Input: part model. Units: mm. Frame: model coordinates. A direction names the side the tool comes from. Give positions to 0.01 mm unless a question says otherwise; leave off trailing zeros. Loops run counter-clockwise (first coordinate to the right, second up) from the corner with the lowest first, then second, coordinate; pieces in that order, holes last. Notation, with made-up numbers: (80.5, -7) -> (139.5, -7) arc R30 cw to (139.5, 24) -> close; hole circle Ø6 at (87.5, 62.5). An arc over 180 degrees is marked (long way). Answer as a JSON object with one key per item and string values.
```python
from build123d import *

# Parameters (mm, degrees)
F0_W     = 50
F0_H     = 100
F1_DEPTH = 2
F2_W     = 8
F2_H     = 20
F3_DEPTH = 10
F4_W     = 4
F4_H     = 36.223298
F5_DEPTH = 10


with BuildPart() as f1:
    # F0 (on Front) → F1 (new body)
    with BuildSketch(Plane.XZ):
        Rectangle(F0_W, F0_H)
    extrude(amount=F1_DEPTH)

    # F2 (on face) → F3 (join)
    with BuildSketch(Plane(origin=(0, 0, 0), x_dir=(-1, 0, 0), z_dir=(0, 1, 0))):
        Rectangle(F2_W, F2_H)
    extrude(amount=F3_DEPTH)

    # F4 (on face) → F5 (cut)
    with BuildSketch(Plane(origin=(0, 10, 0), x_dir=(-1, 0, 0), z_dir=(0, 1, 0))):
        Rectangle(F4_W, F4_H)
    extrude(amount=-F5_DEPTH, mode=Mode.SUBTRACT)


solid = f1.part
```
Q1. Section C-C, the plane x = -9. Return the cut outline in (y, z).
Evaluation:
{"outline": "(-2, -50) -> (0, -50) -> (0, 50) -> (-2, 50) -> close"}
Q2. Section A-A, the plane y = 7.5. Return the cut outline in (x, z).
Evaluation:
{"outline": "(-4, -10) -> (-2, -10) -> (-2, 10) -> (-4, 10) -> close; (2, -10) -> (4, -10) -> (4, 10) -> (2, 10) -> close"}
Q3. Access query for faces 4 (the flat face through (-3, 5, -10)), 5 (the flat face through (-4, 5, 0)), 6 (the flat face through (3, 5, 10)), 7 (the flat face through (4, 5, 0)), 8 (the flat face through (2, 5, 0)). Directions: +Z, -Z, +X, -X, +Y, -Y. A direction counts if a zero-diameter tool reaches every point of the face in a straight line with its end or side. Return the directions, or none.
Evaluation:
{"face 4": "-Z, +X, -X, +Y", "face 5": "+Z, -Z, -X, +Y", "face 6": "+Z, +X, -X, +Y", "face 7": "+Z, -Z, +X, +Y", "face 8": "+Z, -Z, +Y"}
Q4. Ray query, line 1 along X through (y, z) = (9.25, 3.5); line 2 along Y through (x, z) = (-7, -16); line 3 along Z through (x, y) = (-3.5, 8.5). Return the intervals inside material, ascending.
Evaluation:
{"line 1": "x = -4 to -2, 2 to 4", "line 2": "y = -2 to 0", "line 3": "z = -10 to 10"}
Q5. Section B-B, the plane z = 0. Return the cut outline in (x, y), then the cut area to 3 significant figures.
Evaluation:
{"outline": "(-25, -2) -> (25, -2) -> (25, 0) -> (4, 0) -> (4, 10) -> (2, 10) -> (2, 0) -> (-2, 0) -> (-2, 10) -> (-4, 10) -> (-4, 0) -> (-25, 0) -> close", "area": "140 mm2"}
Q6. Section D-D, the plane z = -38. Return the cut outline in (x, y), then the cut area to 3 significant figures.
Evaluation:
{"outline": "(-25, -2) -> (25, -2) -> (25, 0) -> (-25, 0) -> close", "area": "100 mm2"}
Q7. Pin query (flat end, axial travel): pin 1 (1 mm diameter, centred on y = 8.5, z = 4.5, fed in from -X); pin 2 (5 mm diameter, centred on x = -13.5, z = 1, fed in from +Y); pin 3 (0.6 mm diameter, centred on x = -2.5, y = 3.5, fed in from -Z); pin 4 (4 mm diameter, centred on x = -11.5, y = 1, fed in from +Z). Return the tip coordinate at first contact, or that it passes through.
Evaluation:
{"pin 1": "stops at x = -4", "pin 2": "stops at y = 0", "pin 3": "stops at z = -10", "pin 4": "stops at z = 50"}
Q8. Draft query along X for faces 1 (the flat face through (25, -1, -1)), 2 (the flat face through (3, 5, -10)), 3 (the flat face through (-2, 5, 0)). Return one class per face: +X half, -X half, draft (parallel to the pull), parting line (faces both ways), or undercut.
Evaluation:
{"face 1": "+X half", "face 2": "draft", "face 3": "undercut"}
